from build123d import *

# Parameters (mm, degrees)
CROQUIS1_R              = 1.5
SALIENTE_EXTRUIR1_DEPTH = 5
SALIENTE_EXTRUIR2_DEPTH = 6
CORTAR_EXTRUIR2_DEPTH   = 22


with BuildPart() as part:
    # Croquis1 → Saliente-Extruir1 (new body)
    with BuildSketch(Plane(origin=(0, 0, 0), x_dir=(1, 0, 0), z_dir=(0, 1, 0))):
        with BuildLine():
            Line((175, 3), (0, 3))
            ThreePointArc((0, 3), (-3, 0), (0, -3))
            Line((0, -3), (175, -3))
            ThreePointArc((175, -3), (178, 0), (175, 3))
        make_face()
        with Locations(Location((0, 0, 0), (0, 0, 270))):
            Circle(CROQUIS1_R, mode=Mode.SUBTRACT)
        with Locations(Location((175, 0, 0), (0, 0, 270))):
            Circle(CROQUIS1_R, mode=Mode.SUBTRACT)
    extrude(amount=SALIENTE_EXTRUIR1_DEPTH)

    # Croquis2 → Saliente-Extruir2 (add)
    with BuildSketch(Plane(origin=(0, 0, -3), x_dir=(-1, 0, 0), z_dir=(0, 0, -1))):
        Polygon((-132.006982503, 5), (-123.830535375, 13), (-6.765193463, 13), (-2.840646017, 5), (-120, 5), align=None)
    extrude(amount=-SALIENTE_EXTRUIR2_DEPTH)

    # Croquis4 → Cortar-Extruir2 (cut)
    with BuildSketch(Plane(origin=(0, 0, -3), x_dir=(-1, 0, 0), z_dir=(0, 0, -1))):
        Polygon((-9.88159135, 8), (-3.108751036, -5.80610714), (-63.338491444, -7.280350793), (-136.266049088, -6.162343586), (-121.791342394, 8), align=None)
    extrude(amount=-CORTAR_EXTRUIR2_DEPTH, mode=Mode.SUBTRACT)


solid = part.part
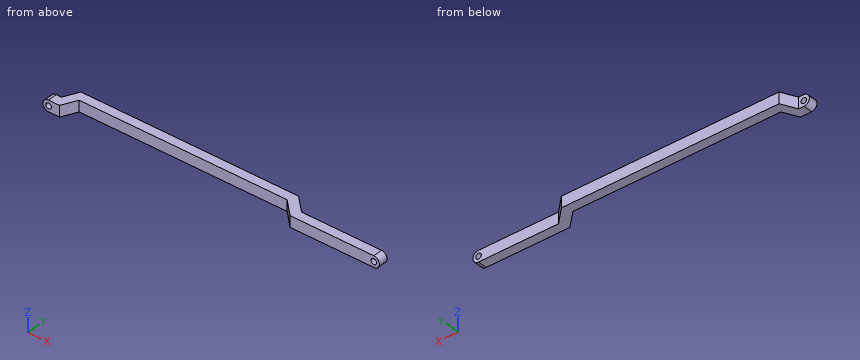
Input: part model. Units: mm. Frame: model coordinates. Round coordinates to 2 decimals unless told otherwise and drop trailing zeros. Write each loop counter-clockwise with the first axis right and the second up, starting at its lowest first coordinate (ties: lowest second). Pieces come first, ordered by that corner, then holes.
1) Cut plane B-B (x = 78.5). Return the cut outline in (y, z).
2) Ray query, L1, parallel to X at y = 3.65, z = 0; L2, parallel to X at y = 4.75, z = -0.5; L3, parallel to Y at x = 40, z = 2.75. Return the intervals inside material, ascending.
3) Cut plane C-C (y = 9.5). Return the cut outline in (x, z).
4) Contact query for flat-ended pins moving along their axis: P1, Ø1, axis at y = 3.5, z = 1.5, coming from the +X side; P2, Ø1.8, axis at x = 0, z = 0, coming from the -Y side; P3, Ø3, axis at x = 62, z = -1, coming from the -Y side. Output: stop coordinate, or through.
5) Cut plane A-A (z = 0). Return the cut outline in (x, y).
Geometry says:
1. outline: (8, -3) - (13, -3) - (13, 3) - (8, 3) - close
2. L1: x = -3 to -1.5, 1.5 to 7.75, 126.24 to 173.5, 176.5 to 178
2. L2: x = -2.96 to -1.41, 1.41 to 8.29, 125.11 to 173.59, 176.41 to 177.96
2. L3: y = 8 to 13
3. outline: (5.05, -3) - (127.41, -3) - (127.41, 3) - (5.05, 3) - close
4. P1: stops at x = 177.83
4. P2: passes through
4. P3: stops at y = 8
5. outline: (-3, 0) - (-1.5, 0) - (-1.5, 5) - (-3, 5) - close; (1.5, 0) - (5.96, 0) - (9.88, 8) - (121.79, 8) - (129.97, 0) - (173.5, 0) - (173.5, 5) - (132.01, 5) - (123.83, 13) - (6.77, 13) - (2.84, 5) - (1.5, 5) - close; (176.5, 0) - (178, 0) - (178, 5) - (176.5, 5) - close
